Part model, mm, in its own coordinate system. Round coordinates to 2 decimals unless told otherwise and drop trailing zeros. Order: outer loops, then holes, each group sorted by start corner. A loop starts at its lowest first (then second) coordinate and runs counter-clockwise, first axis right, second up. Notation, with made-up numbers: (21, 9) - (73, 9) arc R13 cw to (73, 27) - close; hole circle Ø9 at (15, 40). An arc over 180 degrees is marked (long way). Answer as a JSON object with one key per item and string values.
```python
from build123d import *

# Parameters (mm, degrees)
SKETCH_1_W          = 300
SKETCH_1_H          = 220
EXTRUDE_1_DEPTH     = 1
HOLE_WIZARD_M5_1_D  = 5.5
SKETCH_4_W          = 300
SKETCH_4_H          = 20
CUT_EXTRUDE_1_DEPTH = 10
SKETCH_5_R          = 22.5
SKETCH_5_R_2        = 15
SKETCH_5_R_3        = 3.5
CUT_EXTRUDE_2_DEPTH = 10


with BuildPart() as part:
    # 스케치1 → 보스-돌출1 (new body)
    with BuildSketch(Plane.XY):
        Rectangle(SKETCH_1_W, SKETCH_1_H)
    extrude(amount=EXTRUDE_1_DEPTH)

    # M5 여유 구멍1 (through all)
    with Locations(Plane(origin=(0, 0, 0), x_dir=(-1, 0, 0), z_dir=(0, 0, -1))):
        with Locations((-140, 100), (-70, 100), (70, 100), (0, 100), (140, 100), (140, 50), (140, -50), (140, 0), (140, -100), (-140, 50), (-140, -50), (-140, 0), (-140, -100), (-70, -100), (70, -100), (0, -100)):
            Hole(HOLE_WIZARD_M5_1_D / 2)

    # 스케치4 → 컷-돌출1 (cut)
    with BuildSketch(Plane.XY.offset(1)):
        with Locations((0, 100)):
            Rectangle(SKETCH_4_W, SKETCH_4_H)
    extrude(amount=-CUT_EXTRUDE_1_DEPTH, mode=Mode.SUBTRACT)

    # 스케치5 → 컷-돌출2 (cut)
    with BuildSketch(Plane.XY.offset(1)):
        with Locations((-67.5, -25)):
            Circle(SKETCH_5_R)
        with Locations((82.5, -25)):
            Circle(SKETCH_5_R_2)
        with Locations((-25, -47.5)):
            Circle(SKETCH_5_R_3)
        with Locations((-25, -2.5)):
            Circle(SKETCH_5_R_3)
        with Locations((-110, -47.5)):
            Circle(SKETCH_5_R_3)
        with Locations((-110, -2.5)):
            Circle(SKETCH_5_R_3)
    extrude(amount=-CUT_EXTRUDE_2_DEPTH, mode=Mode.SUBTRACT)


solid = part.part
```
Item 1: Cut at A-A (x = -110). Write the cut outline in (y, z).
Taken from the geometry:
{"outline": "(-110, 0) - (-51, 0) - (-51, 1) - (-110, 1) - close; (-44, 0) - (-6, 0) - (-6, 1) - (-44, 1) - close; (1, 0) - (90, 0) - (90, 1) - (1, 1) - close"}
Item 2: Cut at D-D (x = -58). Write the cut outline in (y, z), plus the area to 3 significant figures.
Taken from the geometry:
{"outline": "(-110, 0) - (-45.4, 0) - (-45.4, 1) - (-110, 1) - close; (-4.6, 0) - (90, 0) - (90, 1) - (-4.6, 1) - close", "area": "159 mm2"}
Item 3: Probe L1, parallel to Y at x = 140, z = 0.5; L2, parallel to Y at x = -66, z = 0.85; L3, parallel to Y at x = -23.5, z = 0.5. List the from-to ranges inside material, lowest first. Write a range as from..to.
Taken from the geometry:
{"L1": "-110..-102.75, -97.25..-52.75, -47.25..-2.75, 2.75..47.25, 52.75..90", "L2": "-110..-47.45, -2.55..90", "L3": "-110..-50.66, -44.34..-5.66, 0.66..90"}
Item 4: Cut at C-C (z = 0.45). State how many separate pieces and enclosed holes the cut face has, plus the area to 3 significant figures.
Taken from the geometry:
{"separate pieces": "1", "enclosed holes": "17", "area": "57,300 mm2"}
Item 5: Cut at B-B (y = -25). Write the cut outline in (x, z), plus the area to 3 significant figures.
Taken from the geometry:
{"outline": "(-150, 0) - (-90, 0) - (-90, 1) - (-150, 1) - close; (-45, 0) - (67.5, 0) - (67.5, 1) - (-45, 1) - close; (97.5, 0) - (150, 0) - (150, 1) - (97.5, 1) - close", "area": "225 mm2"}
Item 6: Drop a flat-ended pin along its axis: P1, Ø5.5, axis at x = -25, y = -47.5, coming from the -Z side. Give the stop position or say it passes through.
Taken from the geometry:
{"P1": "through"}
Item 7: Two-plate mould, pull along Y, no slides. Class faces 1 (the flat face through (-2, -9, 1)), 2 (the cylindrical face through (-137.38, 0.83, 0.51)): pulls with the +Y half, pulls with the -Y half, needs draft (parallel to the pull), parting line crosses it, or undercut.
Taken from the geometry:
{"face 1": "needs draft", "face 2": "undercut"}
